Model file for the job. Use its own axes, mm. A direction names the side the tool comes from. Round coordinates to 2 decimals unless told otherwise and drop trailing zeros. Loops run counter-clockwise (first coordinate to the right, second up) from the corner with the lowest first, then second, coordinate; pieces in that order, holes last. Notation, with made-up numbers: M 51,49 L 60,49 A12 ccw 60,67 Z; hole C 56.5,14.5 d1. An arc over 180 degrees is marked long. Answer in a Markdown table with one row per item.
from build123d import *

# Parameters (mm, degrees)
SKETCH3_R          = 6
CUT_EXTRUDE1_DEPTH = 5
SKETCH4_R          = 6
CUT_EXTRUDE2_DEPTH = 5
FILLET1_R          = 1
CHAMFER1_SIZE      = 0.5
CHAMFER1_SIZE2     = 0.575875553


with BuildPart() as part:
    # Sketch1 → Revolve1 (revolve)
    with BuildSketch(Plane.XY, mode=Mode.PRIVATE) as revolve1_sk:
        with BuildLine():
            Line((0, 0), (0, 11.5))
            Line((0, 11.5), (0.5, 12))
            Line((0.5, 12), (2, 12))
            ThreePointArc((2, 12), (2.707106781, 11.707106781), (3, 11))
            Line((3, 11), (3, 10))
            Line((3, 10), (8.07179677, 10))
            ThreePointArc((8.07179677, 10), (8.72645044, 9.755928946), (9.061540088, 9.142857143))
            ThreePointArc((9.061540088, 9.142857143), (10.921361567, 5.599464972), (14.595561276, 4.013646409))
            Line((14.595561276, 4.013646409), (37, 2.5))
            Line((37, 2.5), (37, 8))
            Line((37, 8), (45, 9))
            Line((45, 9), (45, 0))
            Line((45, 0), (0, 0))
        make_face()
    revolve(revolve1_sk.sketch.rotate(Axis((0, 0, 0), (1, 0, 0)), 90), axis=Axis((0, 0, 0), (1, 0, 0)))  # turned: the seam where the file's is

    # Sketch2 → Cut-Revolve1 (revolve, cut)
    with BuildSketch(Plane.XY, mode=Mode.PRIVATE) as cut_revolve1_sk:
        Polygon((4.979432949, 10), (5.5, 9), (6.020567051, 10), align=None)
    revolve(cut_revolve1_sk.sketch.rotate(Axis((0, 0, 0), (1, 0, 0)), 90), axis=Axis((0, 0, 0), (1, 0, 0)), mode=Mode.SUBTRACT)  # turned: the seam where the file's is

    # Sketch3 → Cut-Extrude1 (cut)
    with BuildSketch(Plane.ZY):
        with Locations(Location((0, 0, 0), (0, 0, 270))):  # turned: the seam where the file's is
            Circle(SKETCH3_R)
    extrude(amount=-CUT_EXTRUDE1_DEPTH, mode=Mode.SUBTRACT)

    # Sketch4 → Cut-Extrude2 (cut)
    with BuildSketch(Plane(origin=(45, 0, 0), x_dir=(0, 0, -1), z_dir=(1, 0, 0))):
        with Locations(Location((0, 0, 0), (0, 0, 270))):  # turned: the seam where the file's is
            Circle(SKETCH4_R)
    extrude(amount=-CUT_EXTRUDE2_DEPTH, mode=Mode.SUBTRACT)

    # Fillet1
    fillet1_edges = [part.edges().sort_by_distance(p)[0] for p in [
        (45, 0, -9),
    ]]
    fillet(fillet1_edges, radius=FILLET1_R)

    # Chamfer1
    chamfer1_edges = [part.edges().sort_by_distance(p)[0] for p in [
        (37, 0, -8),
    ]]
    chamfer1_side = [part.faces().sort_by_distance(p)[0] for p in [
        (40.437982633, 0, -8.429747829),
    ]]
    chamfer(chamfer1_edges, length=CHAMFER1_SIZE, length2=CHAMFER1_SIZE2, reference=chamfer1_side[0])


solid = part.part
1. Saw through at A-A (x = 28). Write the cut outline in (y, z).
Verdict:
| item | result |
|---|---|
| outline | C 0,0 d6.22 |
2. Pin check, flat tips, straight feed: pin 1 (5 mm diameter, centred on x = 22.5, z = -3, fed in from -Y); pin 2 (8 mm diameter, centred on x = 14.5, z = 7, fed in from -Y); pin 3 (2 mm diameter, centred on x = 33, y = 0, fed in from -Z). Stop position of each tip, or through.
Verdict:
| item | result |
|---|---|
| pin 1 | stops at y = -3.48 |
| pin 2 | stops at y = -2.86 |
| pin 3 | stops at z = -2.84 |
3. Mould opens along X. For faces 4 (the cylindrical face through (1.26, -3.604, 11.446)), 5 (the flat face through (0, 5, -5)), 6 (the flat face through (40, 0, 0)), 7 (the conical face through (25.955, -0.975, 3.096)) say: +X half, -X half, draft (parallel to the pull), parting line (faces both ways), or undercut.
Verdict:
| item | result |
|---|---|
| face 4 | draft |
| face 5 | -X half |
| face 6 | +X half |
| face 7 | undercut |
4. Wall check: probe 1 along X at (y, z) = (-2.5, 10.25); probe 2 along X at (y, z) = (-8, -5.5); probe 3 along X at (y, z) = (-6.5, -4). Give the ranges that are in metal, low to high.
Verdict:
| item | result |
|---|---|
| probe 1 | x = 0 to 3 |
| probe 2 | x = 0 to 5.13, 5.87 to 8.78 |
| probe 3 | x = 0 to 9.49, 37.16 to 45 |
5. Tool access for faces 1 (the flat face through (3, 10, 2)), 2 (the flat face through (37, 0, -3)), 3 (the flat face through (5, 0, 0)): list every direction of +Z, -Z, +X, -X, +Y, -Y with a clear straight run to the whole face (end or side of a thin tool).
Verdict:
| item | result |
|---|---|
| face 1 | +X |
| face 2 | none |
| face 3 | -X |
